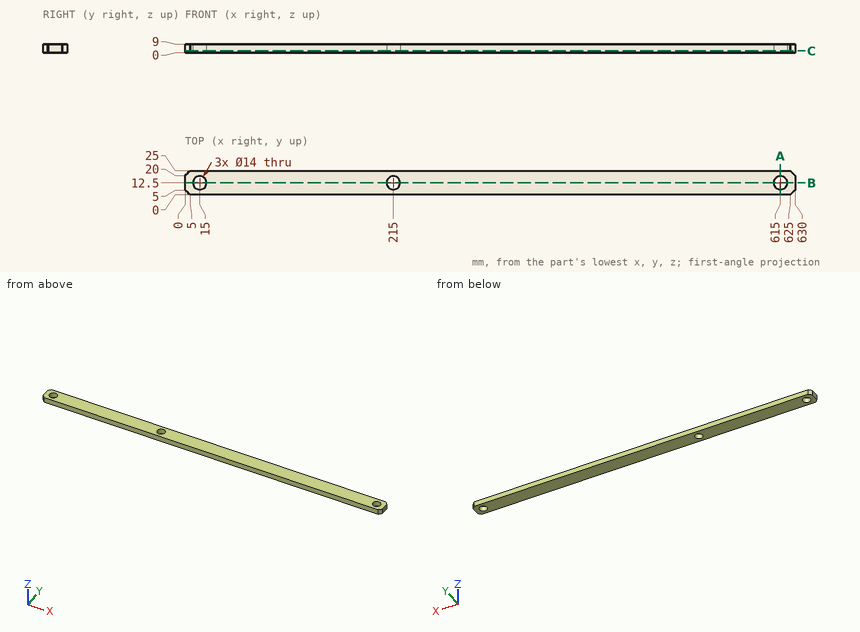
Print and shaded views of the part. All mm, measured from the part's lowest x, y and z. Coordinates: 2 decimals unless noted, no trailing zeros. Loops run counter-clockwise (first coordinate to the right, second up) from the corner with the lowest first, then second, coordinate; pieces in that order, holes last. Notation, with made-up numbers: (53.25, 81.25) - (90.25, 81.25) arc R15 ccw to (90.25, 100.25) - close; hole circle Ø8 at (-28, -30.5). An arc over 180 degrees is marked (long way). Write item = value, one per line. Start each with the question number.
Item 1: Flat gauge pin, fed straight in: pin 1 Ø8.5 at (x, y) = (215, 12.5) entering from +Z. Where does the tip first touch, or does it go through?
Item 2: Wall check: L1, parallel to Y at x = 615, z = 2.5; L2, parallel to X at y = 8, z = 3; L3, parallel to X at y = 6.5, z = 3. Give the ranges that are in metal, low to high. Write a range as from..to.
Item 3: Cut at B-B, the plane y = 12.5. Give the cut face in (x, z), and give its area (3 significant figures).
Item 4: Cut at C-C, the plane z = 2. Give the cut face in (x, y), and give its area (3 significant figures).
Item 5: Cut at A-A, the plane x = 615. Give the cut face in (y, z).
The answers:
q1.pin_1 = through
q2.L1 = 0..5.5, 19.5..25
q2.L2 = 0..9.64, 20.36..209.64, 220.36..609.64, 620.36..630
q2.L3 = 0..11.39, 18.61..211.39, 218.61..611.39, 618.61..630
q3.outline = (0, 0) - (8, 0) - (8, 9) - (0, 9) - close; (22, 0) - (208, 0) - (208, 9) - (22, 9) - close; (222, 0) - (608, 0) - (608, 9) - (222, 9) - close; (622, 0) - (630, 0) - (630, 9) - (622, 9) - close
q3.area = 5,290 mm2
q4.outline = (0, 5) - (5, 0) - (625, 0) - (630, 5) - (630, 20) - (625, 25) - (5, 25) - (0, 20) - close; hole circle Ø14 at (15, 12.5); hole circle Ø14 at (215, 12.5); hole circle Ø14 at (615, 12.5)
q4.area = 15,200 mm2
q5.outline = (0, 0) - (5.5, 0) - (5.5, 9) - (0, 9) - close; (19.5, 0) - (25, 0) - (25, 9) - (19.5, 9) - close
